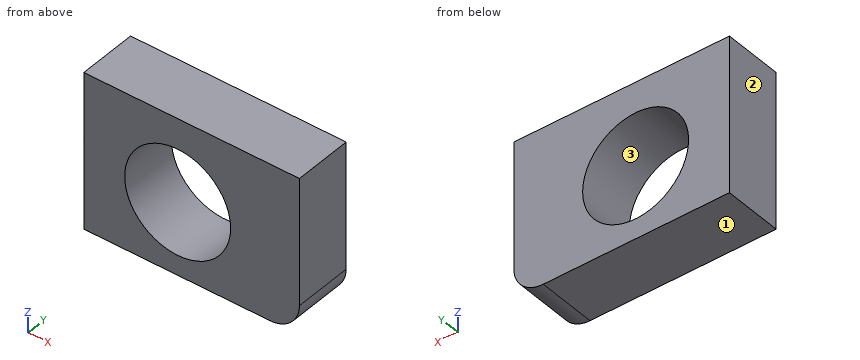
from build123d import *

# Parameters (mm, degrees)
F0_W     = 93.024962
F0_H     = 67.451157
F2_DEPTH = 25.4
F3_R     = 12.7
F4_R     = 22.855993
F5_DEPTH = 25.4


with BuildPart() as f2:
    # F0 (on Front) → F2 (new body)
    with BuildSketch(Plane.XZ):
        with Locations((46.512481, -33.725578)):
            Rectangle(F0_W, F0_H)
    extrude(amount=F2_DEPTH)

    # F3
    f3_edges = [f2.edges().sort_by_distance(p)[0] for p in [
        (93.024962, -12.7, -67.451157),
    ]]
    fillet(f3_edges, radius=F3_R)

    # F4 (on face) → F5 (cut)
    with BuildSketch(Plane.XZ):
        with Locations((40.479131, -36.015701)):
            Circle(F4_R)
    extrude(amount=F5_DEPTH, mode=Mode.SUBTRACT)


solid = f2.part
Source: CAD feature listing. Evaluate the final solid. Frame: model axes, mm. Face numbers are marked on the shaded views. Round coordinates to 2 decimals unless told otherwise and drop trailing zeros. Loops run counter-clockwise (first coordinate to the right, second up) from the corner with the lowest first, then second, coordinate; pieces in that order, holes last. Notation, with made-up numbers: M 68.25,58 L 104.25,58 A15 ccw 104.25,79 Z; hole C 32.5,79 d6. An arc over 180 degrees is marked long. Answer as CSV lines item,"result".
Q1. Contact query for a flat-ended pin moving along its axis: pin 1 (4 mm diameter, centred on y = -18.5, z = -28, fed in from -X). Output: stop coordinate, or through.
Verdict:
pin 1,"stops at x = 0"
Q2. Cut plane A-A (z = -52). Return the cut outline in (x, y), plus the area to 3 significant figures.
Verdict:
outline,"M 0,-25.4 L 24.14,-25.4 L 24.14,0 L 0,0 Z; M 56.82,-25.4 L 93.02,-25.4 L 93.02,0 L 56.82,0 Z"
area,"1,530 mm^2"
Q3. Cut plane B-B (x = 30). Return the cut outline in (y, z), plus the area to 3 significant figures.
Verdict:
outline,"M -25.4,-67.45 L 0,-67.45 L 0,-56.33 L -25.4,-56.33 Z; M -25.4,-15.7 L 0,-15.7 L 0,0 L -25.4,0 Z"
area,"681 mm^2"
Q4. Line query: line 1 along X through (y, z) = (-14, -56); line 2 along Z through (x, y) = (38, -21); line 3 along Z through (x, y) = (33, -9.25). Output: solid intervals per line, ascending.
Verdict:
line 1,"x = 0 to 29.39, 51.57 to 92.96"
line 2,"z = -67.45 to -58.74, -13.29 to 0"
line 3,"z = -67.45 to -57.61, -14.42 to 0"
Q5. Cut plane D-D (z = -61.5). Return the cut outline in (x, y), plus the area to 3 significant figures.
Verdict:
outline,"M 0,-25.4 L 91.08,-25.4 L 91.08,0 L 0,0 Z"
area,"2,310 mm^2"
Q6. Pull-direction query (Z, two-part tool) for the marked faces 1, 2 and 3; classes: +Z half, -Z half, draft (parallel to the pull), parting line (faces both ways), or undercut.
Verdict:
face 1,"-Z half"
face 2,"draft"
face 3,"undercut"
Q7. Cut plane C-C (y = -8). Return the cut outline in (x, z), plus the area to 3 significant figures.
Verdict:
outline,"M 0,-67.45 L 80.32,-67.45 A12.7 ccw 93.02,-54.75 L 93.02,0 L 0,0 Z; hole C 40.48,-36.02 d45.71"
area,"4,600 mm^2"
